from build123d import *

# Parameters (mm, degrees)
SKETCH2_R               = 9.525
SKETCH2_R_2             = 7.112
CUT_EXTRUDE2_DEPTH      = 542
CUT_EXTRUDE2_DEPTH_BACK = 70
SKETCH4_R               = 4
CUT_EXTRUDE3_DEPTH      = 105
CUT_EXTRUDE3_DEPTH_BACK = 311
SKETCH5_R               = 15.875


with BuildPart() as part:
    # Sweep1: sweep along a path in Sketch1
    with BuildLine(Plane.XY) as sweep1_path:
        Line((0, 0), (-117.317574699, 203.2))
    # Sketch2 → Sweep1 (sweep)
    with BuildSketch(Plane(origin=(0, 0, 0), x_dir=(0, 0, 1), z_dir=(-0.5000000000000041, 0.8660254037844362, 0))):
        Circle(SKETCH2_R)
        Circle(SKETCH2_R_2, mode=Mode.SUBTRACT)
    sweep(path=sweep1_path.line)

    # Sketch4 → Cut-Extrude2 (cut, two sides: drawn at the far end of the back side and taken through both)
    with BuildSketch(Plane(origin=(0, 0, 0), x_dir=(1, 0, 0), z_dir=(0, 1, 0)).offset(-CUT_EXTRUDE2_DEPTH_BACK)):
        with Locations(Location((-25.4, 0, 0), (0, 0, 90))):
            Circle(SKETCH4_R)
        with Locations(Location((-91.92, 0, 0), (0, 0, 90))):
            Circle(SKETCH4_R)
    extrude(amount=CUT_EXTRUDE2_DEPTH + CUT_EXTRUDE2_DEPTH_BACK, mode=Mode.SUBTRACT)

    # Sketch5 → Cut-Extrude3 (cut, two sides: drawn at the far end of the back side and taken through both)
    with BuildSketch(Plane(origin=(0, 0, 0), x_dir=(0, 0, -1), z_dir=(1, 0, 0)).offset(-CUT_EXTRUDE3_DEPTH_BACK)):
        with Locations((0, -12)):
            Circle(SKETCH5_R)
        with Locations((0, 215.9625)):
            Circle(SKETCH5_R)
    extrude(amount=CUT_EXTRUDE3_DEPTH + CUT_EXTRUDE3_DEPTH_BACK, mode=Mode.SUBTRACT)


solid = part.part
Geometry: final body of the model. Coordinates: model frame, mm. Give positions to 0.01 mm unless a question says otherwise; leave off trailing zeros. Write each loop counter-clockwise with the first axis right and the second up, starting at its lowest first coordinate (ties: lowest second). Pieces come first, ordered by that corner, then holes.
(1) Mould query, pull axis X, two halves, no side actions, for faces 1 (the flat face through (-123.57, 199.59, -1.46)), 2 (the cylindrical face through (-62.64, 101.2, 8.8)), 3 (the cylindrical face through (-92, 144, -4)), 4 (the flat face through (7.1, 4.1, 0)). Classes: released by +X, released by -X, zero draft, split by the parting line, or undercut.
(2) Ray query, line 1 (X direction, y = 131, z = -2); line 2 (X direction, y = 92, z = 1.75); line 3 (Y direction, x = -40, z = 4.5). Return the intervals inside material, ascending.
(3) First-contact query: P1, Ø1.5, axis at x = -101, z = -0.5, coming from the +Y side; P2, Ø6, axis at x = -106.5, z = -4, coming from the +Y side; P3, Ø7, axis at x = -25.4, z = 0, coming from the +Y side; P4, Ø3, axis at y = 136, z = 6.5, coming from the +X side. Flat tips, straight axial feed; report the tip coordinate or a pass-through.
(4) Cut plane A-A, the plane z = 0. Return loops of the section in (x, y) (1 decimal), then the cut area to 3 significant figures.
Values follow:
1. face 1: released by -X
1. face 2: split by the parting line
1. face 3: undercut
1. face 4: released by +X
2. line 1: x = -86.39 to -83.51, -67.75 to -64.88
2. line 2: x = -63.93 to -61.08, -45.16 to -42.3
2. line 3: y = 52.49 to 58.27, 80.3 to 86.07
3. P1: stops at y = 195.26
3. P2: stops at y = 201.46
3. P3: passes through
3. P4: stops at x = -68.86
4. outline: (-125.6, 198.4) - (-95.9, 147.1) - (-95.9, 151.9) - (-123.5, 199.6) - close; (-107.3, 200.1) - (-95.9, 180.4) - (-95.9, 185.2) - (-104.5, 200.1) - close; (-87.9, 133.2) - (-29.4, 31.9) - (-29.4, 36.7) - (-87.9, 138.1) - close; (-87.9, 166.5) - (-29.4, 65.1) - (-29.4, 70) - (-87.9, 171.3) - close; (-21.4, 18) - (-13.2, 3.9) - (-10.4, 3.9) - (-21.4, 22.8) - close; (-21.4, 51.3) - (6, 3.9) - (6.7, 3.9) - (8.2, 4.8) - (-21.4, 56.1) - close
4. area: 935 mm2
